The listing builds one solid part. Answer for the finished solid, in the listing's coordinates (mm). A direction names the side the tool comes from. Give positions to 0.01 mm unless a question says otherwise; leave off trailing zeros. Order: outer loops, then holes, each group sorted by start corner. A loop starts at its lowest first (then second) coordinate and runs counter-clockwise, first axis right, second up. Notation, with made-up numbers: (27, 35) - (33, 35) arc R16 ccw to (33, 53) - close; hole circle Ø5 at (25, 17.25). An arc over 180 degrees is marked (long way). Use CSV: the item, a comma, the result in double quotes.
```python
from build123d import *

# Parameters (mm, degrees)
F0_W     = 600
F0_H     = 25
F1_DEPTH = 1000
F2_R     = 25
F3_DEPTH = 875
F4_W     = 600
F4_H     = 25
F5_DEPTH = 1000


with BuildPart() as f1:
    # F0 (on Front) → F1 (new body)
    with BuildSketch(Plane.XZ):
        with Locations((300, 887.5)):
            Rectangle(F0_W, F0_H)
    extrude(amount=F1_DEPTH)

    # F2 (on face) → F3 (join)
    with BuildSketch(Plane(origin=(0, 0, 875), x_dir=(1, 0, 0), z_dir=(0, 0, -1))):
        with Locations((525, 75)):
            Circle(F2_R)
        with Locations((62.72, 75)):
            Circle(F2_R)
        with Locations((525, 943.68)):
            Circle(F2_R)
        with Locations((62.72, 943.68)):
            Circle(F2_R)
    extrude(amount=F3_DEPTH)

    # F4 (on face) → F5 (join)
    with BuildSketch(Plane(origin=(0, 0, 0), x_dir=(-1, 0, 0), z_dir=(0, 1, 0))):
        with Locations((-300, 462.5)):
            Rectangle(F4_W, F4_H)
    extrude(amount=-F5_DEPTH)


solid = f1.part
```
Item 1: The part is cut by section A-A (x = 525). Give the vertices of the cut face in (y, z).
Taken from the geometry:
outline,"(-1000, 450) - (-968.68, 450) - (-968.68, 0) - (-918.68, 0) - (-918.68, 450) - (-100, 450) - (-100, 0) - (-50, 0) - (-50, 450) - (0, 450) - (0, 475) - (-50, 475) - (-50, 875) - (0, 875) - (0, 900) - (-1000, 900) - (-1000, 875) - (-968.68, 875) - (-968.68, 475) - (-1000, 475) - close; hole (-918.68, 475) - (-100, 475) - (-100, 875) - (-918.68, 875) - close"
Item 2: The part is cut by section B-B (y = -767.5). Give the vertices of the cut face in (x, z), and give its area (3 significant figures).
Taken from the geometry:
outline,"(0, 450) - (600, 450) - (600, 475) - (0, 475) - close; (0, 875) - (600, 875) - (600, 900) - (0, 900) - close"
area,"30,000 mm^2"
Item 3: The part is cut by section D-D (y = -943.68). Give the vertices of the cut face in (x, z), and give its area (3 significant figures).
Taken from the geometry:
outline,"(0, 450) - (37.72, 450) - (37.72, 0) - (87.72, 0) - (87.72, 450) - (500, 450) - (500, 0) - (550, 0) - (550, 450) - (600, 450) - (600, 475) - (550, 475) - (550, 875) - (600, 875) - (600, 900) - (0, 900) - (0, 875) - (37.72, 875) - (37.72, 475) - (0, 475) - close; hole (87.72, 475) - (500, 475) - (500, 875) - (87.72, 875) - close"
area,"115,000 mm^2"
Item 4: The mould has two halves that part along Z. Classify faces 4 (the face through (304, -1000, 463)), 5 (the face through (304, -493, 450)), 6 (the face through (57.3, -919.274, 677.8)): +Z half, -Z half, draft (parallel to the pull), parting line (faces both ways), or undercut.
Taken from the geometry:
face 4,"draft"
face 5,"-Z half"
face 6,"undercut"
Item 5: The part is cut by section C-C (z = 700). Give the vertices of the cut face in (x, y), and give its area (3 significant figures).
Taken from the geometry:
outline,"circle Ø50 at (62.72, -943.68); circle Ø50 at (62.72, -75); circle Ø50 at (525, -943.68); circle Ø50 at (525, -75)"
area,"7,850 mm^2"
Item 6: Which of the six approach directions +Z, -Z, +X, -X, +Y, -Y give full straight-line access (tool end or side, diameter ignored) to faces 1 (the face through (85.81, -65.42, 228.15)), 2 (the face through (548.846, -82.509, 677.8)), 3 (the face through (600, -493, 462))?
Taken from the geometry:
face 1,"-Z"
face 2,"none"
face 3,"+Z, -Z, +X, +Y, -Y"
Item 7: This flat-tipped pin is pushed along its axis until it touches: pin 1 (8 mm diameter, centred on x = 103.5, y = -732, fed in from -Z). Where does it stop, or does it pass through?
Taken from the geometry:
pin 1,"z = 450"
Item 8: Find the intervals of material crossed by line 1 along Z through (x, y) = (313, -310); line 2 along Y through (x, z) = (525, 139.5); line 3 along Y through (x, z) = (59, 178), in increasing order.
Taken from the geometry:
line 1,"450 to 475, 875 to 900"
line 2,"-968.68 to -918.68, -100 to -50"
line 3,"-968.4 to -918.96, -99.72 to -50.28"
